from build123d import *

# Parameters (mm, degrees)
SKETCH_W        = 108
SKETCH_H        = 75.2
SKETCH_R        = 1.55
PAD_DEPTH       = 4
SKETCH001_R     = 3.05
POCKET_DEPTH    = 2
POCKET001_DEPTH = 2.5
SKETCH003_R     = 1.55
POCKET002_DEPTH = 4


with BuildPart() as part:
    # Sketch → Pad (new body)
    with BuildSketch(Plane.XY):
        Rectangle(SKETCH_W, SKETCH_H)
        with Locations((-10, 10)):
            Circle(SKETCH_R, mode=Mode.SUBTRACT)
        with Locations((10, 10)):
            Circle(SKETCH_R, mode=Mode.SUBTRACT)
        with Locations((10, -10)):
            Circle(SKETCH_R, mode=Mode.SUBTRACT)
        with Locations((-10, -10)):
            Circle(SKETCH_R, mode=Mode.SUBTRACT)
    extrude(amount=PAD_DEPTH)

    # Sketch001 (on Face10 of Pad) → Pocket (cut)
    with BuildSketch(Plane.XY.offset(4)):
        with Locations((-15, 15)):
            Circle(SKETCH001_R)
        with Locations((15, 15)):
            Circle(SKETCH001_R)
        with Locations((15, -15)):
            Circle(SKETCH001_R)
        with Locations((-15, -15)):
            Circle(SKETCH001_R)
    extrude(amount=-POCKET_DEPTH, mode=Mode.SUBTRACT)

    # Sketch002 (on Face5 of Pocket) → Pocket001 (cut)
    with BuildSketch(Plane.XY.offset(4)):
        Polygon((-47, 31.645448), (-47, 34.936345), (-49.85, 36.581793), (-52.7, 34.936345), (-52.7, 31.645448), (-49.85, 30), align=None)
        Polygon((-49.85, -36.581793), (-47, -34.936345), (-47, -31.645448), (-49.85, -30), (-52.7, -31.645448), (-52.7, -34.936345), align=None)
        Polygon((52.7, -34.936345), (52.7, -31.645448), (49.85, -30), (47, -31.645448), (47, -34.936345), (49.85, -36.581793), align=None)
        Polygon((52.7, 31.645448), (52.7, 34.936345), (49.85, 36.581793), (47, 34.936345), (47, 31.645448), (49.85, 30), align=None)
        Polygon((-36.65, 22.854552), (-36.65, 26.145448), (-39.5, 27.790897), (-42.35, 26.145448), (-42.35, 22.854552), (-39.5, 21.209103), align=None)
        Polygon((21.35, 26.145448), (18.5, 27.790897), (15.65, 26.145448), (15.65, 22.854552), (18.5, 21.209103), (21.35, 22.854552), align=None)
        Polygon((21.35, -26.145448), (21.35, -22.854552), (18.5, -21.209103), (15.65, -22.854552), (15.65, -26.145448), (18.5, -27.790897), align=None)
        Polygon((-36.65, -26.145448), (-36.65, -22.854552), (-39.5, -21.209103), (-42.35, -22.854552), (-42.35, -26.145448), (-39.5, -27.790897), align=None)
    extrude(amount=-POCKET001_DEPTH, mode=Mode.SUBTRACT)

    # Sketch003 (on Face5 of Pocket001) → Pocket002 (cut)
    with BuildSketch(Plane.XY.offset(4)):
        with Locations((-49.75, 33.291)):
            Circle(SKETCH003_R)
        with Locations((-39.5, 24.5)):
            Circle(SKETCH003_R)
        with Locations((18.5, 24.5)):
            Circle(SKETCH003_R)
        with Locations((49.75, 33.291)):
            Circle(SKETCH003_R)
        with Locations((49.75, -33.291)):
            Circle(SKETCH003_R)
        with Locations((18.5, -24.5)):
            Circle(SKETCH003_R)
        with Locations((-39.5, -24.5)):
            Circle(SKETCH003_R)
        with Locations((-49.75, -33.291)):
            Circle(SKETCH003_R)
    extrude(amount=-POCKET002_DEPTH, mode=Mode.SUBTRACT)


solid = part.part
Could you check a few things on this model? Use its own coordinates, in mm. A direction names the side the tool comes from. Coordinates: 2 decimals unless noted, no trailing zeros. Order: outer loops, then holes, each group sorted by start corner. A loop starts at its lowest first (then second) coordinate and runs counter-clockwise, first axis right, second up. Notation, with made-up numbers: (-16.5, -34) -> (37.5, -34) arc R19 cw to (37.5, -16) -> close; hole circle Ø4 at (-30.5, -38.75). An arc over 180 degrees is marked (long way). One line per item, written item: value. Start each with the question number.
1) Which directions (+Z, -Z, +X, -X, +Y, -Y) give clear straight access to the entire face, cutting with the end or side of a thin tool? Please do faces 5 (the cylindrical face through (18.298, -22.963, 0.76)), 6 (the flat face through (-51.255, -30.811, 2.768)).
2) Imagine slicing it at A-A on y = 24.5. List the corners of the cut face in (x, z) for me, plus the area to 3 significant figures.
3) I'm going to push flat-ended pins straight in: pin 1 (4 mm diameter, centred on x = 49.75, y = -33.291, fed in from +Z); pin 2 (2.5 mm diameter, centred on x = 10, y = -10, fed in from +Z). Where does each tip first touch, or does it pass through?
4) Imagine slicing it at C-C on y = -15. List the corners of the cut face in (x, z) for me.
5) Imagine slicing it at B-B on x = -10. List the corners of the cut face in (y, z) for me, plus the area to 3 significant figures.
6) If I drill on L1, parallel to Y at x = -15, z = 3.5; L2, parallel to Y at x = -39.5, z = 0.55; L3, parallel to X at y = -32.5, z = 1.75, over which ranges is the centre line in solid material (lowest first)? Write a range as [from, to].
7) Imagine slicing it at D-D on y = 10. List the corners of the cut face in (x, z) for me.
8) We'd pull the mould along Y, two halves only. Please class faces 1 (the flat face through (50, -35, 1.5)), 2 (the flat face through (-1, -37.6, 2)), 3 (the flat face through (-54, -1, 2)), 4 (the flat face through (47, -33, 3)): +Y half, -Y half, draft (parallel to the pull), parting line (faces both ways), or undercut.
Answer list:
1. face 5: +Z, -Z
1. face 6: +Z
2. outline: (-54, 0) -> (-41.05, 0) -> (-41.05, 1.5) -> (-42.35, 1.5) -> (-42.35, 4) -> (-54, 4) -> close; (-37.95, 0) -> (16.95, 0) -> (16.95, 1.5) -> (15.65, 1.5) -> (15.65, 4) -> (-36.65, 4) -> (-36.65, 1.5) -> (-37.95, 1.5) -> close; (20.05, 0) -> (54, 0) -> (54, 4) -> (21.35, 4) -> (21.35, 1.5) -> (20.05, 1.5) -> close
2. area: 394 mm2
3. pin 1: stops at z = 1.5
3. pin 2: passes through
4. outline: (-54, 0) -> (54, 0) -> (54, 4) -> (18.05, 4) -> (18.05, 2) -> (11.95, 2) -> (11.95, 4) -> (-11.95, 4) -> (-11.95, 2) -> (-18.05, 2) -> (-18.05, 4) -> (-54, 4) -> close
5. outline: (-37.6, 0) -> (-11.55, 0) -> (-11.55, 4) -> (-37.6, 4) -> close; (-8.45, 0) -> (8.45, 0) -> (8.45, 4) -> (-8.45, 4) -> close; (11.55, 0) -> (37.6, 0) -> (37.6, 4) -> (11.55, 4) -> close
5. area: 276 mm2
6. L1: y = [-37.6, -18.05], [-11.95, 11.95], [18.05, 37.6]
6. L2: y = [-37.6, -26.05], [-22.95, 22.95], [26.05, 37.6]
6. L3: x = [-54, -52.7], [-47, 47], [52.7, 54]
7. outline: (-54, 0) -> (-11.55, 0) -> (-11.55, 4) -> (-54, 4) -> close; (-8.45, 0) -> (8.45, 0) -> (8.45, 4) -> (-8.45, 4) -> close; (11.55, 0) -> (54, 0) -> (54, 4) -> (11.55, 4) -> close
8. face 1: undercut
8. face 2: -Y half
8. face 3: draft
8. face 4: undercut
